```python
from build123d import *

# Parameters (mm, degrees)
SKETCH1_W           = 2400
SKETCH1_H           = 1200
SKETCH1_R           = 60
BOSS_EXTRUDE1_DEPTH = 18
BOSS_EXTRUDE2_START = 18
SKETCH2_W           = 600
SKETCH2_H           = 1200
BOSS_EXTRUDE2_DEPTH = 68
SKETCH3_R           = 10
SKETCH3_R_2         = 9
BOSS_EXTRUDE3_DEPTH = 300
SKETCH4_R           = 10
SKETCH4_R_2         = 9
BOSS_EXTRUDE4_DEPTH = 150
SKETCH6_R           = 6
BOSS_EXTRUDE5_DEPTH = 5
SKETCH7_R           = 6
BOSS_EXTRUDE6_DEPTH = 5


with BuildPart() as part:
    # Sketch1 → Boss-Extrude1 (new body)
    with BuildSketch(Plane(origin=(0, 0, 0), x_dir=(1, 0, 0), z_dir=(0, 1, 0))):
        Rectangle(SKETCH1_W, SKETCH1_H)
        with Locations(Location((0, -443.053648657, 0), (0, 0, 270))):
            Circle(SKETCH1_R, mode=Mode.SUBTRACT)
    extrude(amount=BOSS_EXTRUDE1_DEPTH)

    # Sketch2 → Boss-Extrude2 (add)
    with BuildSketch(Plane(origin=(0, 0, 0), x_dir=(1, 0, 0), z_dir=(0, 1, 0)).offset(BOSS_EXTRUDE2_START)):
        with Locations((-900, 0)):
            Rectangle(SKETCH2_W, SKETCH2_H)
        with Locations((900, 0)):
            Rectangle(SKETCH2_W, SKETCH2_H)
    extrude(amount=BOSS_EXTRUDE2_DEPTH)

    # Sketch3 → Boss-Extrude3 (add)
    with BuildSketch(Plane(origin=(0, 86, 0), x_dir=(1, 0, 0), z_dir=(0, 1, 0))):
        with Locations(Location((-800, 0, 0), (0, 0, 270))):
            Circle(SKETCH3_R)
        with Locations(Location((-800, 0, 0), (0, 0, 270))):
            Circle(SKETCH3_R_2, mode=Mode.SUBTRACT)
    extrude(amount=BOSS_EXTRUDE3_DEPTH)

    # Sketch4 → Boss-Extrude4 (add)
    with BuildSketch(Plane(origin=(0, 86, 0), x_dir=(1, 0, 0), z_dir=(0, 1, 0))):
        with Locations(Location((750, 0, 0), (0, 0, 270))):
            Circle(SKETCH4_R)
        with Locations(Location((750, 0, 0), (0, 0, 270))):
            Circle(SKETCH4_R_2, mode=Mode.SUBTRACT)
    extrude(amount=BOSS_EXTRUDE4_DEPTH)

    # Sketch6 → Boss-Extrude5 (add)
    # profile 1 of 2: a face of its own
    with BuildSketch(Plane(origin=(0, 86, 0), x_dir=(1, 0, 0), z_dir=(0, 1, 0))):
        Polygon((-800, -512.227333668), (-789.410818423, -506.113666834), (-789.410818423, -493.886333166), (-800, -487.772666332), (-810.589181577, -493.886333166), (-810.589181577, -506.113666834), align=None)
        with Locations(Location((-800, -500, 0), (0, 0, 270))):
            Circle(SKETCH6_R, mode=Mode.SUBTRACT)
    # profile 2 of 2: a face of its own
    with BuildSketch(Plane(origin=(0, 86, 0), x_dir=(1, 0, 0), z_dir=(0, 1, 0))):
        Polygon((-900, 360.617779526), (-909.195266801, 355.308889763), (-909.195266801, 344.691110237), (-900, 339.382220474), (-890.804733199, 344.691110237), (-890.804733199, 355.308889763), align=None)
        with Locations(Location((-900, 350, 0), (0, 0, 270))):
            Circle(SKETCH6_R, mode=Mode.SUBTRACT)
    extrude(amount=BOSS_EXTRUDE5_DEPTH)

    # Sketch7 → Boss-Extrude6 (add)
    # profile 1 of 2: a face of its own
    with BuildSketch(Plane(origin=(0, 86, 0), x_dir=(1, 0, 0), z_dir=(0, 1, 0))):
        Polygon((750, -410.254981665), (758.881074637, -405.127490833), (758.881074637, -394.872509167), (750, -389.745018335), (741.118925363, -394.872509167), (741.118925363, -405.127490833), align=None)
        with Locations(Location((750, -400, 0), (0, 0, 270))):
            Circle(SKETCH7_R, mode=Mode.SUBTRACT)
    # profile 2 of 2: a face of its own
    with BuildSketch(Plane(origin=(0, 86, 0), x_dir=(1, 0, 0), z_dir=(0, 1, 0))):
        Polygon((800, 460.50831519), (790.899532094, 455.254157595), (790.899532094, 444.745842405), (800, 439.49168481), (809.100467906, 444.745842405), (809.100467906, 455.254157595), align=None)
        with Locations(Location((800, 450, 0), (0, 0, 270))):
            Circle(SKETCH7_R, mode=Mode.SUBTRACT)
    extrude(amount=BOSS_EXTRUDE6_DEPTH)


solid = part.part
```
Build history of the part. All positions in model axes, mm. A direction names the side the tool comes from. Round coordinates to 2 decimals unless told otherwise and drop trailing zeros. Order: outer loops, then holes, each group sorted by start corner. A loop starts at its lowest first (then second) coordinate and runs counter-clockwise, first axis right, second up. Notation, with made-up numbers: (6, 44) -> (47, 44) arc R24 cw to (47, 66) -> close; hole circle Ø8 at (74.25, 85). An arc over 180 degrees is marked (long way). Answer in a Markdown table with one row per item.
1) Band-saw the part on C-C on x = 271. Give the cut face in (y, z), and give its area (3 significant figures).
Values:
| item | result |
|---|---|
| outline | (0, -600) -> (18, -600) -> (18, 600) -> (0, 600) -> close |
| area | 21,600 mm2 |
2) Which spindle directions (+Z, -Z, +X, -X, +Y, -Y) get a long thin tool onto all of the face, cutting with end or side? Do faces 1 (the flat face through (600, 52, 8)), 2 (the flat face through (-17, 14, 600)). Say none if no direction does.
Values:
| item | result |
|---|---|
| face 1 | +Z, -Z, +Y |
| face 2 | +Z, +X, -X, +Y, -Y |
3) Band-saw the part on D-D on x = 973. Give the cut face in (y, z).
Values:
| item | result |
|---|---|
| outline | (0, -600) -> (86, -600) -> (86, 600) -> (0, 600) -> close |
4) Pin check, flat tips, straight feed: P1, Ø5.5, axis at y = 87.5, z = -448, coming from the +X side; P2, Ø9.5, axis at x = -799.5, z = 502.5, coming from the +Y side; P3, Ø6, axis at x = 745, z = -3, coming from the +Y side; P4, Ø3, axis at x = 36, z = -206.5, coming from the +Y side. Stop position of each tip, or through.
Values:
| item | result |
|---|---|
| P1 | x = 1200 |
| P2 | y = 91 |
| P3 | y = 86 |
| P4 | y = 18 |
5) Wall check: L1, parallel to X at y = 88.9, z = 500; L2, parallel to X at y = 87, z = 400; L3, parallel to X at y = 194, z = 0. Give the ranges that are in metal, low to high.
Values:
| item | result |
|---|---|
| L1 | -810.59 to -806, -794 to -789.41 |
| L2 | 741.12 to 744, 756 to 758.88 |
| L3 | -810 to -809, -791 to -790, 740 to 741, 759 to 760 |
6) Band-saw the part on B-B on z = -114. Give the cut face in (x, y), and give its area (3 significant figures).
Values:
| item | result |
|---|---|
| outline | (-1200, 0) -> (1200, 0) -> (1200, 86) -> (600, 86) -> (600, 18) -> (-600, 18) -> (-600, 86) -> (-1200, 86) -> close |
| area | 125,000 mm2 |
7) Mould opens along X. For faces 3 (the flat face through (-17, 14, -600)), 4 (the flat face through (-600, 52, 8)), 5 (the flat face through (-1200, 42, 8)) say: released by +X, released by -X, zero draft, split by the parting line, or undercut.
Values:
| item | result |
|---|---|
| face 3 | zero draft |
| face 4 | undercut |
| face 5 | released by -X |
8) Band-saw the part on A-A on y = 120.5. Give the cut face in (x, z).
Values:
| item | result |
|---|---|
| outline | circle Ø20 at (-800, 0); circle Ø20 at (750, 0); hole circle Ø18 at (-800, 0); hole circle Ø18 at (750, 0) |
